```python
from build123d import *

# Parameters (mm, degrees)
BOSS_EXTRUDE1_DEPTH     = 19
CUT_EXTRUDE1_DEPTH      = 49.249947637
CUT_EXTRUDE1_DEPTH_BACK = 109.67350832


with BuildPart() as part:
    # Sketch1 → Boss-Extrude1 (new body)
    with BuildSketch(Plane.XY):
        with BuildLine():
            Line((-265.157990376, 195.999066862), (-226.911895103, 162.718581948))
            ThreePointArc((-226.911895103, 162.718581948), (-269.236431055, 159.780273509), (-266.298122616, 117.455737558))
            Line((-266.298122616, 117.455737558), (-304.54421789, 150.736222472))
            ThreePointArc((-304.54421789, 150.736222472), (-331.112603464, 213.622868622), (-265.157990376, 195.999066862))
        make_face()
        with BuildLine():
            Line((-300.79209478, 160.727155027), (-282.314825505, 144.648847504))
            ThreePointArc((-282.314825505, 144.648847504), (-273.762715494, 163.71889626), (-256.057340496, 174.824077098))
            Line((-256.057340496, 174.824077098), (-274.534609771, 190.902384621))
            ThreePointArc((-274.534609771, 190.902384621), (-323.568796066, 207.05849737), (-300.79209478, 160.727155027))
        make_face(mode=Mode.SUBTRACT)
    extrude(amount=BOSS_EXTRUDE1_DEPTH)

    # Sketch2 → Cut-Extrude1 (cut, two sides)
    with BuildSketch(Plane(origin=(-17.199721271, -19.766003413, 0), x_dir=(0.75438074, -0.656437125, 0), z_dir=(0.656437125, 0.75438074, 0))) as cut_extrude1_sk:
        with BuildLine():
            Line((-407.026362297, 14.142127452), (-297.992481459, 14.142127452))
            Line((-297.992481459, 14.142127452), (-297.992481459, 0))
            ThreePointArc((-297.992481459, 0), (-313.1180692, -4.209672376), (-328.716129113, -6))
            Line((-328.716129113, -6), (-407.026362297, -6))
            Line((-407.026362297, -6), (-407.026362297, 14.142127452))
        make_face()
    extrude(amount=CUT_EXTRUDE1_DEPTH, mode=Mode.SUBTRACT)
    extrude(cut_extrude1_sk.sketch, amount=-CUT_EXTRUDE1_DEPTH_BACK, mode=Mode.SUBTRACT)


solid = part.part
```
CAD build for the part. Positions are in the model's coordinates, mm. A direction names the side the tool comes from. Give positions to 0.01 mm unless a question says otherwise; leave off trailing zeros. Loops run counter-clockwise (first coordinate to the right, second up) from the corner with the lowest first, then second, coordinate; pieces in that order, holes last. Notation, with made-up numbers: M 19,-26 L 30,-26 A25 cw 30,4 Z; hole C -18,77.25 d2. An arc over 180 degrees is marked long. Use one line per item in the form item = value.
Item 1: Which spindle directions (+Z, -Z, +X, -X, +Y, -Y) get a long thin tool onto all of the face, cutting with end or side? Do faces 5 (the face through (-322.954, 207.742, 12.409)), 6 (the face through (-327, 203, 6)). Say none if no direction does.
Determined:
face_5 = +Z, -Z
face_6 = -Z, -X, +Y
Item 2: Slice it at A-A (z = 10.75). List the corners of the cut face in (x, y) (3 decimals).
Determined:
outline = M -304.544,150.736 L -266.298,117.456 A30 cw -226.912,162.719 L -265.158,195.999 A38 ccw long Z; hole M -300.792,160.727 L -282.315,144.649 A36 cw -256.057,174.824 L -274.535,190.902 A28 ccw long Z
Item 3: Drill centre lines: probe 1 along Y at (x, z) = (-292.5, 8); probe 2 along X at (y, z) = (165.5, 12.25) (3 decimals); probe 3 along Y at (x, z) = (-288, 13.25). Where is each one in solid material? Low to high. Write a range as from..to.
Determined:
probe_1 = 140.26..153.51, 214.85..225.35
probe_2 = -332.559..-318.155, -272.104..-262.548, -230.662..-230.108
probe_3 = 136.34..149.6, 212.66..223.83
Item 4: Slice it at B-B (y = 128). List the corners of the cut face in (x, z).
Determined:
outline = M -278.42,0 L -274.06,0 L -274.06,19 L -278.42,19 Z
Item 5: Flat gauge pins, fed straight in: pin 1 (22.5 mm diameter, centred on x = -312, y = 177.5, fed in from -Z); pin 2 (5 mm diameter, centred on y = 156, z = 6, fed in from -X); pin 3 (10 mm diameter, centred on x = -269.5, y = 193, fed in from -Z); pin 4 (6 mm diameter, centred on y = 145.5, z = 13.5, fed in from +X). Where does each tip first touch, or does it go through?
Determined:
pin_1 = through
pin_2 = -325.54
pin_3 = 5.8
pin_4 = -275.4
Item 6: Two-plate mould, pull along Y, no slides. Class faces 1 (the face through (-272.664, 163.32, 4.167)), 2 (the face through (-285.15, 133.86, 11.48)), 3 (the face through (-265.167, 182.751, 12.686)), 4 (the face through (-291.68, 152.8, 12.69)): pulls with the +Y half, pulls with the -Y half, needs draft (parallel to the pull), parting line crosses it, or undercut.
Determined:
face_1 = pulls with the +Y half
face_2 = pulls with the -Y half
face_3 = undercut
face_4 = undercut
